Geometry check sheet. Reference: the model listing, model coordinates, mm. Give positions to 0.01 mm unless a question says otherwise; leave off trailing zeros. Write item = value, one per line. Start each with the question number.
(1) Thickness scan on L1, parallel to X at y = 17.5, z = -168; L2, parallel to Y at x = -15, z = -182. Record the ranges inside material, lowest first.
(2) Section check A-A, the plane z = 80. Give the number of separate pieces and of enclosed holes in the cut face, plus the area to 3 significant figures.
(3) Depth check by flat-ended pin: pin 1 Ø0.8 at (x, z) = (-19.5, -123) entering from +Y; pin 2 Ø0.5 at (x, z) = (-5.5, -59) entering from -Y. Enter the tip coordinate at first touch or a pass-through.
(4) Draft check along X on faces 1 (the flat face through (18.25, -15, -48)), 2 (the flat face through (20, 11, -48)). Enter one of: pulls with the +X half, pulls with the -X half, needs draft (parallel to the pull), parting line crosses it, or undercut.
```python
from build123d import *

# Parameters (mm, degrees)
BOSS_EXTRU_1_DEPTH = 300


with BuildPart() as part:
    # Esquisse1 → Boss.-Extru.1 (new body)
    with BuildSketch(Plane.XY.offset(100)):
        with BuildLine():
            Line((6, -19), (6, -20))
            Line((6, -20), (17, -20))
            ThreePointArc((17, -20), (19.121320344, -19.121320344), (20, -17))
            Line((20, -17), (20, -6))
            Line((20, -6), (19, -6))
            Line((19, -6), (19, -5))
            Line((19, -5), (16, -5))
            Line((16, -5), (16, -10))
            Line((16, -10), (11.697056276, -10))
            Line((11.697056276, -10), (6.44138072, -4.744324444))
            ThreePointArc((6.44138072, -4.744324444), (7.551143817, -2.642011933), (7.994130058, -0.306405969))
            Line((7.994130058, -0.306405969), (7.7, 0))
            Line((7.7, 0), (7.994130058, 0.306405971))
            ThreePointArc((7.994130058, 0.306405971), (7.551143817, 2.642011934), (6.441380719, 4.744324444))
            Line((6.441380719, 4.744324444), (11.697056275, 10))
            Line((11.697056275, 10), (16, 10))
            Line((16, 10), (16, 5))
            Line((16, 5), (19, 5))
            Line((19, 5), (19, 6))
            Line((19, 6), (20, 6))
            Line((20, 6), (20, 17))
            ThreePointArc((20, 17), (19.121320344, 19.121320344), (17, 20))
            Line((17, 20), (6, 20))
            Line((6, 20), (6, 19))
            Line((6, 19), (5, 19))
            Line((5, 19), (5, 15.999999999))
            Line((5, 15.999999999), (10.000000001, 15.999999999))
            Line((10.000000001, 15.999999999), (10.000000001, 11.697056275))
            Line((10.000000001, 11.697056275), (4.744324444, 6.441380719))
            ThreePointArc((4.744324444, 6.441380719), (2.642011933, 7.551143817), (0.306405969, 7.994130058))
            Line((0.306405969, 7.994130058), (0, 7.7))
            Line((0, 7.7), (-0.30640597, 7.994130058))
            ThreePointArc((-0.30640597, 7.994130058), (-2.642011933, 7.551143817), (-4.744324444, 6.441380719))
            Line((-4.744324444, 6.441380719), (-9.999999999, 11.697056274))
            Line((-9.999999999, 11.697056274), (-9.999999999, 15.999999999))
            Line((-9.999999999, 15.999999999), (-5, 15.999999999))
            Line((-5, 15.999999999), (-5, 19))
            Line((-5, 19), (-6, 19))
            Line((-6, 19), (-6, 20))
            Line((-6, 20), (-17, 20))
            ThreePointArc((-17, 20), (-19.121320344, 19.121320344), (-20, 17))
            Line((-20, 17), (-20, 6))
            Line((-20, 6), (-19, 6))
            Line((-19, 6), (-19, 5))
            Line((-19, 5), (-16, 5))
            Line((-16, 5), (-16, 10))
            Line((-16, 10), (-11.697056274, 10))
            Line((-11.697056274, 10), (-6.441380718, 4.744324445))
            ThreePointArc((-6.441380718, 4.744324445), (-7.551143817, 2.642011933), (-7.994130058, 0.306405969))
            Line((-7.994130058, 0.306405969), (-7.699999999, 0))
            Line((-7.699999999, 0), (-7.994130057, -0.306405971))
            ThreePointArc((-7.994130057, -0.306405971), (-7.551143816, -2.642011934), (-6.441380719, -4.744324444))
            Line((-6.441380719, -4.744324444), (-11.697056275, -10))
            Line((-11.697056275, -10), (-16, -10))
            Line((-16, -10), (-16, -5))
            Line((-16, -5), (-19, -5))
            Line((-19, -5), (-19, -6))
            Line((-19, -6), (-20, -6))
            Line((-20, -6), (-20, -17))
            ThreePointArc((-20, -17), (-19.121320344, -19.121320344), (-17, -20))
            Line((-17, -20), (-6, -20))
            Line((-6, -20), (-6, -19))
            Line((-6, -19), (-5, -19))
            Line((-5, -19), (-5, -16.000000001))
            Line((-5, -16.000000001), (-9.999999999, -16.000000001))
            Line((-9.999999999, -16.000000001), (-9.999999999, -11.697056274))
            Line((-9.999999999, -11.697056274), (-4.744324444, -6.441380719))
            ThreePointArc((-4.744324444, -6.441380719), (-2.642011933, -7.551143817), (-0.306405969, -7.994130058))
            Line((-0.306405969, -7.994130058), (0, -7.7))
            Line((0, -7.7), (0.306405971, -7.994130058))
            ThreePointArc((0.306405971, -7.994130058), (2.642011934, -7.551143817), (4.744324445, -6.441380719))
            Line((4.744324445, -6.441380719), (10.000000001, -11.697056274))
            Line((10.000000001, -11.697056274), (10.000000001, -16.000000001))
            Line((10.000000001, -16.000000001), (5, -16.000000001))
            Line((5, -16.000000001), (5, -19))
            Line((5, -19), (6, -19))
        make_face()
        with BuildLine():
            Line((18.25, 12.25), (12.25, 12.25))
            Line((12.25, 12.25), (12.25, 18.25))
            Line((12.25, 18.25), (17.25, 18.25))
            ThreePointArc((17.25, 18.25), (17.957106781, 17.957106781), (18.25, 17.25))
            Line((18.25, 17.25), (18.25, 12.25))
        make_face(mode=Mode.SUBTRACT)
        with BuildLine():
            Line((-18.25, -12.25), (-12.25, -12.25))
            Line((-12.25, -12.25), (-12.25, -18.25))
            Line((-12.25, -18.25), (-17.25, -18.25))
            ThreePointArc((-17.25, -18.25), (-17.957106781, -17.957106781), (-18.25, -17.25))
            Line((-18.25, -17.25), (-18.25, -12.25))
        make_face(mode=Mode.SUBTRACT)
        with BuildLine():
            Line((-12.25, 18.25), (-12.25, 12.25))
            Line((-12.25, 12.25), (-18.25, 12.25))
            Line((-18.25, 12.25), (-18.25, 17.25))
            ThreePointArc((-18.25, 17.25), (-17.957106781, 17.957106781), (-17.25, 18.25))
            Line((-17.25, 18.25), (-12.25, 18.25))
        make_face(mode=Mode.SUBTRACT)
        with BuildLine():
            Line((12.25, -18.25), (12.25, -12.25))
            Line((12.25, -12.25), (18.25, -12.25))
            Line((18.25, -12.25), (18.25, -17.25))
            ThreePointArc((18.25, -17.25), (17.957106781, -17.957106781), (17.25, -18.25))
            Line((17.25, -18.25), (12.25, -18.25))
        make_face(mode=Mode.SUBTRACT)
        with BuildLine():
            Line((-5.705709703, -4.055228326), (-4.075506937, -2.896591666))
            ThreePointArc((-4.075506937, -2.896591666), (-4.635549589, -1.873947727), (-4.943520622, -0.749402378))
            Line((-4.943520622, -0.749402378), (-5.932224738, -0.899282852))
            ThreePointArc((-5.932224738, -0.899282852), (-6, 0), (-5.932224738, 0.899282853))
            Line((-5.932224738, 0.899282853), (-4.943520622, 0.749402379))
            ThreePointArc((-4.943520622, 0.749402379), (-4.635549588, 1.873947727), (-4.075506937, 2.896591666))
            Line((-4.075506937, 2.896591666), (-5.705709704, 4.055228326))
            ThreePointArc((-5.705709704, 4.055228326), (-4.953610357, 4.945881563), (-4.064132573, 5.699370705))
            Line((-4.064132573, 5.699370705), (-2.902951842, 4.070979081))
            ThreePointArc((-2.902951842, 4.070979081), (-1.877566249, 4.634085136), (-0.749402377, 4.943520623))
            Line((-0.749402377, 4.943520623), (-0.899282852, 5.932224739))
            ThreePointArc((-0.899282852, 5.932224739), (0, 6), (0.899282852, 5.932224739))
            Line((0.899282852, 5.932224739), (0.749402377, 4.943520623))
            ThreePointArc((0.749402377, 4.943520623), (1.87756625, 4.634085136), (2.902951843, 4.07097908))
            Line((2.902951843, 4.07097908), (4.064132575, 5.699370704))
            ThreePointArc((4.064132575, 5.699370704), (4.953610358, 4.945881562), (5.705709704, 4.055228326))
            Line((5.705709704, 4.055228326), (4.075506937, 2.896591666))
            ThreePointArc((4.075506937, 2.896591666), (4.635549589, 1.873947727), (4.943520623, 0.749402378))
            Line((4.943520623, 0.749402378), (5.932224739, 0.899282853))
            ThreePointArc((5.932224739, 0.899282853), (6, 0), (5.932224739, -0.899282853))
            Line((5.932224739, -0.899282853), (4.943520623, -0.749402379))
            ThreePointArc((4.943520623, -0.749402379), (4.635549589, -1.873947727), (4.075506938, -2.896591666))
            Line((4.075506938, -2.896591666), (5.705709704, -4.055228326))
            ThreePointArc((5.705709704, -4.055228326), (4.953610357, -4.945881563), (4.064132573, -5.699370705))
            Line((4.064132573, -5.699370705), (2.902951842, -4.070979081))
            ThreePointArc((2.902951842, -4.070979081), (1.87756625, -4.634085136), (0.749402378, -4.943520623))
            Line((0.749402378, -4.943520623), (0.899282852, -5.932224739))
            ThreePointArc((0.899282852, -5.932224739), (1e-09, -6), (-0.899282851, -5.932224739))
            Line((-0.899282851, -5.932224739), (-0.749402377, -4.943520623))
            ThreePointArc((-0.749402377, -4.943520623), (-1.87756625, -4.634085136), (-2.902951843, -4.07097908))
            Line((-2.902951843, -4.07097908), (-4.064132574, -5.699370704))
            ThreePointArc((-4.064132574, -5.699370704), (-4.953610357, -4.945881562), (-5.705709703, -4.055228326))
        make_face(mode=Mode.SUBTRACT)
    extrude(amount=-BOSS_EXTRU_1_DEPTH)


solid = part.part
```
Model answer:
q1.L1 = -19.96 to -18.22, -12.25 to -5, 5 to 12.25, 18.22 to 19.96
q1.L2 = -20 to -18.25, -12.25 to -10, 10 to 12.25, 18.25 to 20
q2.separate_pieces = 1
q2.enclosed_holes = 5
q2.area = 566 mm²
q3.pin_1 = 19.14
q3.pin_2 = -19
q4.face_1 = undercut
q4.face_2 = pulls with the +X half
